Geometry check sheet. Reference: the model listing, model coordinates, mm. Coordinates: 2 decimals unless noted, no trailing zeros. Write each loop counter-clockwise with the first axis right and the second up, starting at its lowest first coordinate (ties: lowest second). Pieces come first, ordered by that corner, then holes. Notation, with made-up numbers: (15, 86) - (67, 86) arc R30 cw to (67, 117) - close; hole circle Ø1 at (-16, 68). An arc over 180 degrees is marked (long way). Answer as a JSON object with one key per item and string values. Group by question number.
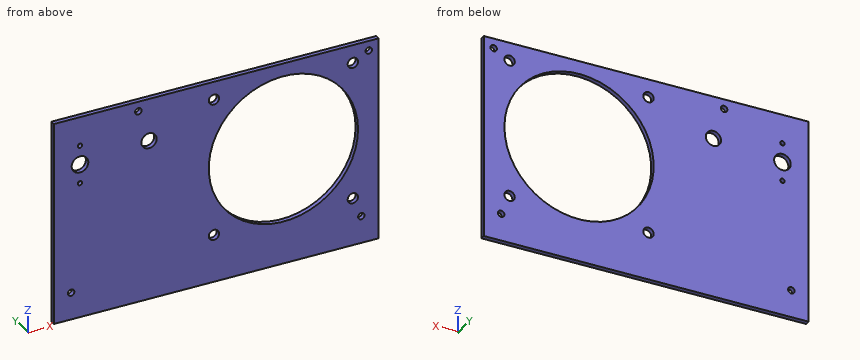
from build123d import *

# Parameters (mm, degrees)
F0_W     = 174
F0_H     = 110
F0_R     = 1.75
F0_R_2   = 2.778
F0_R_3   = 1.2
F0_R_4   = 4.45
F0_R_5   = 4.1
F0_R_6   = 40
F1_DEPTH = 2.5


# Not quite as in the source:
# - a feature names something its author has since deleted; it is built from what else it names


with BuildPart() as f1:
    # F0 (on Front) → F1 (new body)
    with BuildSketch(Plane.XZ):
        Rectangle(F0_W, F0_H)
        with Locations((-77.75, -40.25)):
            Circle(F0_R, mode=Mode.SUBTRACT)
        with Locations((-1.222, -29.222)):
            Circle(F0_R_2, mode=Mode.SUBTRACT)
        with Locations((77.75, -40.25)):
            Circle(F0_R, mode=Mode.SUBTRACT)
        with Locations((73.222, -29.222)):
            Circle(F0_R_2, mode=Mode.SUBTRACT)
        with Locations((-73, 18.7)):
            Circle(F0_R_3, mode=Mode.SUBTRACT)
        with Locations((-73, 29)):
            Circle(F0_R_4, mode=Mode.SUBTRACT)
        with Locations((-73, 39.3)):
            Circle(F0_R_3, mode=Mode.SUBTRACT)
        with Locations((-36, 32)):
            Circle(F0_R_5, mode=Mode.SUBTRACT)
        with Locations((-41.75, 49.75)):
            Circle(F0_R, mode=Mode.SUBTRACT)
        with Locations((-1.222, 45.222)):
            Circle(F0_R_2, mode=Mode.SUBTRACT)
        with Locations((36, 8)):
            Circle(F0_R_6, mode=Mode.SUBTRACT)
        with Locations((73.222, 45.222)):
            Circle(F0_R_2, mode=Mode.SUBTRACT)
        with Locations((81.75, 49.75)):
            Circle(F0_R, mode=Mode.SUBTRACT)
    extrude(amount=F1_DEPTH)


solid = f1.part
(1) Section check A-A (x = 36). Record the cut outline in (y, z).
(2) Section check D-D (y = -0.9). Count the separate pieces of the cut face and the enclosed holes in it, and give its area (3 significant figures).
(3) Gauge pin test, flat end, axial feed: pin 1 (1.4 mm diameter, centred on x = -73, z = 39.3, fed in from +Y). Record the tip position at first contact, or that the pin passes through.
(4) Section check C-C (z = 8). Record the cut outline in (x, y).
(5) Section check B-B (z = 49.75). Record the cut outline in (x, y), and give its area (4 significant figures).
(6) Material ranges on L1, parallel to X at y = -0.9, z = 31; L2, parallel to Z at x = 77.75, y = -1.5; L3, parallel to Z at x = -41.75, y = -0.9, recorded low to high. Write a range as [from, to].
Conclusion:
{
 "1": {"outline": "(-2.5, -55) - (0, -55) - (0, -32) - (-2.5, -32) - close; (-2.5, 48) - (0, 48) - (0, 55) - (-2.5, 55) - close"},
 "2": {"separate pieces": "1", "enclosed holes": "13", "area": "13,900 mm^2"},
 "3": {"pin 1": "passes through"},
 "4": {"outline": "(-87, -2.5) - (-4, -2.5) - (-4, 0) - (-87, 0) - close; (76, -2.5) - (87, -2.5) - (87, 0) - (76, 0) - close"},
 "5": {"outline": "(-87, -2.5) - (-43.5, -2.5) - (-43.5, 0) - (-87, 0) - close; (-40, -2.5) - (80, -2.5) - (80, 0) - (-40, 0) - close; (83.5, -2.5) - (87, -2.5) - (87, 0) - (83.5, 0) - close", "area": "417.5 mm^2"},
 "6": {"L1": "x = [-87, -76.98], [-69.02, -39.98], [-32.02, 3.27], [68.73, 87]", "L2": "z = [-55, -42], [-38.5, 55]", "L3": "z = [-55, 48], [51.5, 55]"}
}
